from build123d import *

# Parameters (mm, degrees)
SKETCH2_R           = 1.5
BOSS_EXTRUDE2_DEPTH = 3


with BuildPart() as part:
    # Sketch2 → Boss-Extrude2 (new body)
    # profile 1 of 2: a face of its own
    with BuildSketch(Plane(origin=(0, 84, 0), x_dir=(1, 0, 0), z_dir=(0, 1, 0))):
        with BuildLine():
            ThreePointArc((-6.349779829, 90.729255992), (-8.48155795, 87.141170391), (-5.66275018, 84.063320655))
            ThreePointArc((-5.66275018, 84.063320655), (-4.641171279, 84.018442382), (-3.65022139, 84.270743452))
            ThreePointArc((-3.65022139, 84.270743452), (-1.51844327, 87.858829053), (-4.33725104, 90.936678789))
            Line((-4.33725104, 90.936678789), (-5.374827195, 91.136771127))
            Line((-5.374827195, 91.136771127), (-6.349779829, 90.729255992))
        make_face()
        with Locations(Location((-5.00000061, 87.499999722, 0), (0, 0, 270))):
            Circle(SKETCH2_R, mode=Mode.SUBTRACT)
    # profile 2 of 2: a face of its own
    with BuildSketch(Plane(origin=(0, 84, 0), x_dir=(1, 0, 0), z_dir=(0, 1, 0))):
        with BuildLine():
            Line((-77.167393969, 97.852700174), (-5.66275018, 84.063320655))
            ThreePointArc((-5.66275018, 84.063320655), (-8.48155795, 87.141170391), (-6.349779829, 90.729255992))
            Line((-6.349779829, 90.729255992), (-5.374827195, 91.136771127))
            Line((-5.374827195, 91.136771127), (-75.841894829, 104.726058307))
            ThreePointArc((-75.841894829, 104.726058307), (-79.941323466, 101.952128811), (-77.167393969, 97.852700174))
        make_face()
        with Locations(Location((-76.504644399, 101.28937924, 0), (0, 0, 270))):
            Circle(SKETCH2_R, mode=Mode.SUBTRACT)
    extrude(amount=BOSS_EXTRUDE2_DEPTH)


solid = part.part
Source: CAD feature listing. Evaluate the final solid. Frame: model axes, mm. Round coordinates to 2 decimals unless told otherwise and drop trailing zeros. Write each loop counter-clockwise with the first axis right and the second up, starting at its lowest first coordinate (ties: lowest second). Pieces come first, ordered by that corner, then holes. Notation, with made-up numbers: (1, -15) - (28, -15) arc R27 cw to (28, 18) - close; hole circle Ø6 at (60, -33.75). An arc over 180 degrees is marked (long way). Use CSV: the item, a comma, the result in double quotes. Start each with the question number.
(1) Cut plane B-B, the plane z = -87.5. Return loops of the section in (x, y), and give its area (3 significant figures).
(2) Mould query, pull axis X, two halves, no side actions, for faces 1 (the face through (-41, 84, -95)), 2 (the face through (-41.916, 85.479, -91.055)), 3 (the face through (-77.835, 85.479, -100.597)). Classes: pulls with the +X half, pulls with the -X half, needs draft (parallel to the pull), parting line crosses it, or undercut.
(3) Cut plane A-A, the plane y = 85.85. Return loops of the section in (x, z).
(4) Cut plane C-C, the plane x = -15. Return loops of the section in (y, z).
(5) First-contact query: pin 1 Ø1.5 at (x, y) = (-36.5, 85) entering from +Z; pin 2 Ø1 at (x, y) = (-40.5, 85) entering from +Z. Flat tips, straight axial feed; report the tip coordinate or a pass-through.
(6) Material intervals for probe 1 along Z at (x, y) = (-5, 85.2); probe 2 along Z at (x, y) = (-11, 86.4); probe 3 along Z at (x, y) = (-23, 86), sorted ascending. Write a range as [from, to].
(7) Cut plane D-D, the plane z = -94.25. Return loops of the section in (x, y).
Geometry says:
1,outline,"(-23.48, 84) - (-6.5, 84) - (-6.5, 87) - (-23.48, 87) - close; (-3.5, 84) - (-1.5, 84) - (-1.5, 87) - (-3.5, 87) - close"
1,area,"57.0 mm²"
2,face 1,"needs draft"
2,face 2,"pulls with the -X half"
2,face 3,"undercut"
3,outline,"(-77.17, -97.85) arc R3.5 ccw to (-75.84, -104.73) - (-4.34, -90.94) arc R3.5 ccw to (-5.66, -84.06) - close; hole circle Ø3 at (-76.5, -101.29); hole circle Ø3 at (-5, -87.5)"
4,outline,"(84, -92.99) - (87, -92.99) - (87, -85.86) - (84, -85.86) - close"
5,pin 1,"z = -89.87"
5,pin 2,"z = -90.69"
6,probe 1,"[-91.06, -89], [-86, -84]"
6,probe 2,"[-92.22, -85.09]"
6,probe 3,"[-94.54, -87.41]"
7,outline,"(-58.49, 84) - (-21.52, 84) - (-21.52, 87) - (-58.49, 87) - close"
